The model under review builds one solid part; all positions refer to its coordinate system, in mm. Coordinates: 2 decimals unless noted, no trailing zeros. Order: outer loops, then holes, each group sorted by start corner. A loop starts at its lowest first (then second) coordinate and runs counter-clockwise, first axis right, second up.
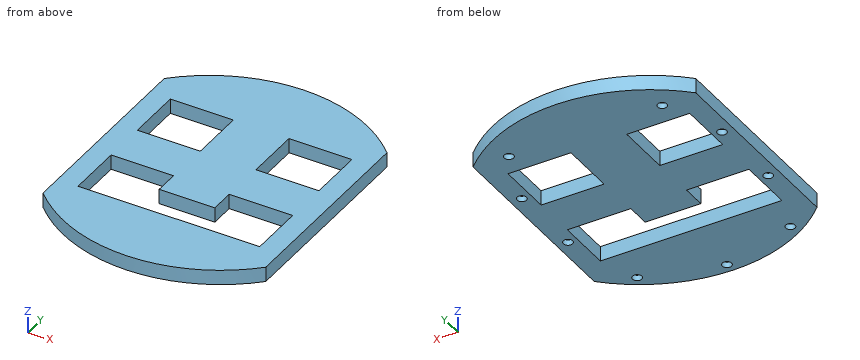
```python
from build123d import *

# Parameters (mm, degrees)
RESSALTO_EXTRUS_O1_DEPTH = 8
CORTE_EXTRUS_O1_DEPTH    = 10
RESSALTO_EXTRUS_O2_REACH = 161.117
ESBO_O3_W                = 30
ESBO_O3_H                = 8
ESBO_O4_R                = 2.5
CORTE_EXTRUS_O2_DEPTH    = 3


with BuildPart() as part:
    # Esboço1 → Ressalto-extrusão1 (new body)
    with BuildSketch(Plane.XY):
        with BuildLine():
            Line((0, 0), (0, -110))
            ThreePointArc((0, -110), (60, -134.792027106), (120, -110))
            Line((120, -110), (120, 0))
            ThreePointArc((120, 0), (60, 24.792027106), (0, 0))
        make_face()
    extrude(amount=RESSALTO_EXTRUS_O1_DEPTH)

    # Esboço2 → Corte-extrusão1 (cut)
    with BuildSketch(Plane(origin=(0, 0, 0), x_dir=(-1, 0, 0), z_dir=(0, 0, -1))):
        Polygon((-108.919644627, -96.875), (-11.080355373, -96.875), (-11.080355373, -66.875), (-44.695581191, -66.875), (-44.695581191, -79.875), (-74.695581191, -79.875), (-74.695581191, -66.875), (-108.919644627, -66.875), align=None)
        Polygon((-108.919644627, -43.125), (-75, -43.125), (-75, -30.608967116), (-45, -30.608967116), (-45, -43.125), (-11.080355373, -43.125), (-11.080355373, -13.125), (-108.919644627, -13.125), align=None)
    extrude(amount=-CORTE_EXTRUS_O1_DEPTH, mode=Mode.SUBTRACT)

    # Esboço3 → Ressalto-extrusão2 (add, up to next)
    with BuildSketch(Plane(origin=(0, -30.608967116, 0), x_dir=(1, 0, 0), z_dir=(0, 1, 0)), mode=Mode.PRIVATE) as ressalto_extrus_o2_sk1:
        with Locations((60, -4)):
            Rectangle(ESBO_O3_W, ESBO_O3_H)
    ressalto_extrus_o2_tool1 = extrude(ressalto_extrus_o2_sk1.sketch, amount=RESSALTO_EXTRUS_O2_REACH, mode=Mode.PRIVATE) - part.part
    add(ressalto_extrus_o2_tool1.solids().sort_by_distance((60, -30.608967, 4))[0])

    # Esboço4 → Corte-extrusão2 (cut)
    with BuildSketch(Plane(origin=(0, 0, 0), x_dir=(-1, 0, 0), z_dir=(0, 0, -1))):
        with Locations((-18.70841508, -1.064839346)):
            Circle(ESBO_O4_R)
        with Locations((-6.09375, -34.065)):
            Circle(ESBO_O4_R)
        with Locations((-6.09375, -75.94)):
            Circle(ESBO_O4_R)
        with Locations((-18.70841508, -117.382967977)):
            Circle(ESBO_O4_R)
        with Locations((-60, -129.382503442)):
            Circle(ESBO_O4_R)
        with Locations((-101.29158492, -117.382967977)):
            Circle(ESBO_O4_R)
        with Locations((-113.90625, -75.94)):
            Circle(ESBO_O4_R)
        with Locations((-113.90625, -34.065)):
            Circle(ESBO_O4_R)
        with Locations((-101.29158492, -1.064839346)):
            Circle(ESBO_O4_R)
    extrude(amount=-CORTE_EXTRUS_O2_DEPTH, mode=Mode.SUBTRACT)


solid = part.part
```
(1) Wall thickness on probe 1 along X at (y, z) = (-36, 3.25); probe 2 along X at (y, z) = (-67, 6.25); probe 3 along Y at (x, z) = (19.5, 6.5) (3 decimals): over which ranges is each line inside the solid? List them lowest first.
A:
probe 1: x = 0 to 11.08, 45 to 75, 108.92 to 120
probe 2: x = 0 to 11.08, 44.7 to 74.7, 108.92 to 120
probe 3: y = -124.523 to -96.875, -66.875 to -43.125, -13.125 to 14.523
(2) We need section C-C, the plane z = 4.25. Write out the cut boundary in (x, y) (3 decimals).
A:
outline: (0, -110) arc R85 ccw to (120, -110) - (120, 0) arc R85 ccw to (0, 0) - close; hole (11.08, -96.875) - (108.92, -96.875) - (108.92, -66.875) - (74.696, -66.875) - (74.696, -79.875) - (44.696, -79.875) - (44.696, -66.875) - (11.08, -66.875) - close; hole (11.08, -43.125) - (45, -43.125) - (45, -13.125) - (11.08, -13.125) - close; hole (75, -43.125) - (108.92, -43.125) - (108.92, -13.125) - (75, -13.125) - close
(3) For pin 1 Ø4 at (x, z) = (43, 6.5) entering from +Y; pin 2 Ø1.5 at (x, y) = (114, -34) entering from -Z; pin 3 Ø2 at (x, z) = (93.5, 6.5) entering from -Y, all flat-tipped, find the tip position at first contact; note any pin that passes through.
A:
pin 1: stops at y = 23.46
pin 2: stops at z = 3
pin 3: stops at y = -128.33
(4) We need section B-B, the plane y = -94. Write out the cut boundary in (x, z).
A:
outline: (0, 0) - (11.08, 0) - (11.08, 8) - (0, 8) - close; (108.92, 0) - (120, 0) - (120, 8) - (108.92, 8) - close
(5) We need section A-A, the plane x = 60. Write out the cut boundary in (y, z) (1 decimal), and give its area (3 significant figures).
A:
outline: (-134.8, 0) - (-131.9, 0) - (-131.9, 3) - (-126.9, 3) - (-126.9, 0) - (-96.9, 0) - (-96.9, 8) - (-134.8, 8) - close; (-79.9, 0) - (24.8, 0) - (24.8, 8) - (-79.9, 8) - close
area: 1,130 mm2
(6) We need section D-D, the plane y = -75.94. Write out the cut boundary in (x, z), and give its area (3 significant figures).
A:
outline: (0, 0) - (3.59, 0) - (3.59, 3) - (8.59, 3) - (8.59, 0) - (11.08, 0) - (11.08, 8) - (0, 8) - close; (44.7, 0) - (74.7, 0) - (74.7, 8) - (44.7, 8) - close; (108.92, 0) - (111.41, 0) - (111.41, 3) - (116.41, 3) - (116.41, 0) - (120, 0) - (120, 8) - (108.92, 8) - close
area: 387 mm2
